Can you work these out from the drawing? Everything is in mm from the part's minimum corner. A direction names the side the tool comes from. Coordinates: 2 decimals unless noted, no trailing zeros. Order: outer loops, then holes, each group sorted by start corner. A loop starts at its lowest first (then second) coordinate and runs counter-clockwise, first axis right, second up. Notation, with made-up numbers: (56.25, 11) - (71.25, 11) arc R14 ccw to (71.25, 36) - close; hole circle Ø5 at (-38, 19). An arc over 180 degrees is marked (long way). Use one line per item in the form item = value. Start each with the question number.
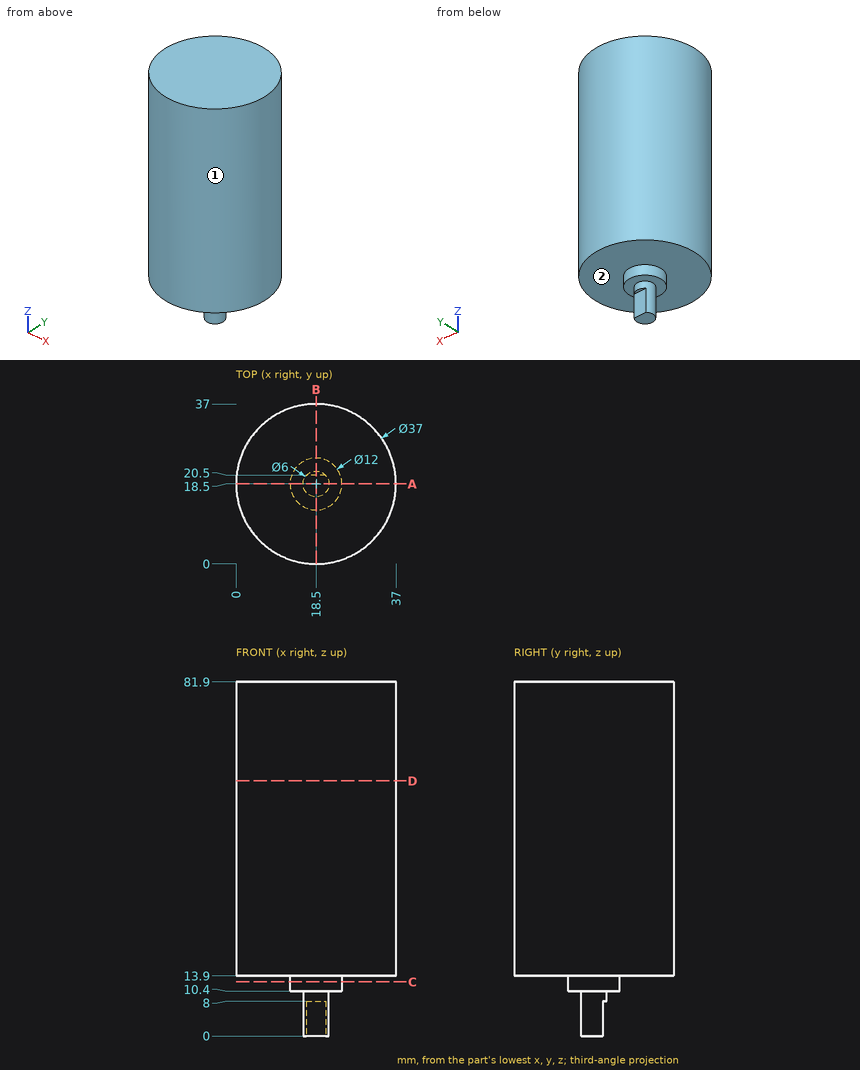
1) For pin 1 (6 mm diameter, centred on x = 23.5, z = 14.5, fed in from +Y); pin 2 (5 mm diameter, centred on x = 19.5, z = 5, fed in from +Y); pin 3 (10 mm diameter, centred on y = 24, z = 56.5, fed in from -X), each with a flat end and sliding along its axis, tell me the tip position at first contact or that it passes through.
2) Suppose I cut it at C-C, the plane z = 12.5. List the corners of the cut face in (x, y) for me.
3) I need wall thicknesses on probe 1 along Z at (x, y) = (10.5, 34); probe 2 along Y at (x, z) = (32.5, 70); probe 3 along X at (y, z) = (2.5, 63). Which ranges of each line are inside material? Lowest first, please. Write a range as [from, to].
4) Suppose I cut it at D-D, the plane z = 59. List the corners of the cut face in (x, y) for me, then the cut area to 3 significant figures.
5) Which directions (+Z, -Z, +X, -X, +Y, -Y) give clear straight access to the entire face, cutting with the end or side of a thin tool? Please do the marked faces 1 and 2.
6) Suppose I cut it at A-A, the plane y = 18.5. List the corners of the cut face in (x, z) for me, then the cut area to 3 significant figures.
7) Suppose I cut it at B-B, the plane x = 18.5. List the corners of the cut face in (y, z) for me.
From the geometry:
q1.pin_1 = 36.89
q1.pin_2 = 20.5
q1.pin_3 = 0.01
q2.outline = circle Ø12 at (18.5, 18.5)
q3.probe_1 = [13.9, 81.9]
q3.probe_2 = [6.41, 30.59]
q3.probe_3 = [9.21, 27.79]
q4.outline = circle Ø37 at (18.5, 18.5)
q4.area = 1,080 mm2
q5.face_1 = +Z, -Z
q5.face_2 = -Z
q6.outline = (0, 13.9) - (12.5, 13.9) - (12.5, 10.4) - (15.5, 10.4) - (15.5, 0) - (21.5, 0) - (21.5, 10.4) - (24.5, 10.4) - (24.5, 13.9) - (37, 13.9) - (37, 81.9) - (0, 81.9) - close
q6.area = 2,620 mm2
q7.outline = (0, 13.9) - (12.5, 13.9) - (12.5, 10.4) - (15.5, 10.4) - (15.5, 0) - (20.5, 0) - (20.5, 8) - (21.5, 8) - (21.5, 10.4) - (24.5, 10.4) - (24.5, 13.9) - (37, 13.9) - (37, 81.9) - (0, 81.9) - close
